Autodesk Inventor part; units mm, degrees
ref_plane "YZ Plane" through (0, 0, 0) normal (1, 0, 0) x (0, 1, 0)
ref_plane "XZ Plane" through (0, 0, 0) normal (0, 1, 0) x (-1, 0, 0)
ref_plane "XY Plane" through (0, 0, 0) normal (0, 0, 1) x (1, 0, 0)
sketch "Sketch1" plane through (0, 0, 0) normal (0, 0, 1) x (1, 0, 0)
  line L0 (0, 8.1389) -> (7.0485, 4.0695)
  line L1 (7.0485, 4.0695) -> (7.0485, -4.0695)
  line L2 (7.0485, -4.0695) -> (0, -8.1389)
  line L3 (0, -8.1389) -> (-7.0485, -4.0695)
  line L4 (-7.0485, -4.0695) -> (-7.0485, 4.0695)
  line L5 (-7.0485, 4.0695) -> (0, 8.1389)
  line L6 (0, 11.3945) -> (0, -11.3945)
  line L7 (-9.8679, 0) -> (9.8679, 0)
  point P0 (0, 0)
  dimension "d0" = 14.097
extrude "Extrusion1" add sketch "Sketch1" along normal blind 11.6332
sketch "Sketch2" plane through (0, 0, 0) normal (1, 0, 0) x (0, 1, 0)
  line L0 (8.1389, 0) -> (8.1389, 11.6332)
  line L1 (4.0695, 11.6332) -> (-4.0695, 11.6332)
  line L2 (8.1389, 11.6332) -> (4.0695, 11.6332)
  line L3 (4.0695, 11.6332) -> (8.1389, 11.6332)
  line L4 (-4.0695, 11.6332) -> (4.0695, 11.6332)
  line L5 (-8.1389, 11.6332) -> (-4.0695, 11.6332)
  line L6 (-4.0695, 11.6332) -> (-8.1389, 11.6332)
  line L7 (8.1389, 7.4422) -> (6.5913, 8.9898)
  line L8 (6.5913, 8.9898) -> (6.5913, 11.6332)
  line L9 (8.1389, 11.6332) -> (8.1389, 7.4422)
  line L10 (6.223, 11.2522) -> (3.683, 11.2522)
  line L11 (3.683, 11.2522) -> (3.683, 8.7122)
  line L12 (3.683, 8.7122) -> (6.223, 8.7122)
  line L13 (6.223, 8.7122) -> (6.223, 11.2522)
  line L14 (0, 18.0282) -> (0, -3.0895)
  arc A0 (7.0485, 0) -> (8.1389, 0.762) centre (6.1895, 2.3903) ccw
  line L15 (8.1389, 0) -> (4.0695, 0)
  line L16 (7.0485, 0) -> (8.1389, 0)
  line L17 (8.1389, 0.762) -> (8.1389, 0)
  dimension "d3" = 4.191
  dimension "d4" = 45
  dimension "d5" = 6.5913
  dimension "d6" = 3.683
  dimension "d7" = 0.381
  dimension "d8" = 2.54
  dimension "d9" = 2.54
  dimension "d11" = 7.0485
  dimension "d12" = 0.762
  dimension "d13" = 2.54
revolve "Revolution1" cut sketch "Sketch2" angle 360 about axis through (0, 0, 0) along (0, 0, -1) contours L7 L8 L2 L0
revolve "Revolution2" cut sketch "Sketch2" angle 360 about axis through (0, 0, 0) along (0, 0, -1) contours L15 A0 L0
hole "Hole1" at (0, 0, 11.6332) direction (0, 0, -1) diameter 7.7978 end through all
fillet "Fillet1" radius 0.381 3 edges at (0, -6.5913, 8.9898) (0, -6.5913, 11.6332) (0, 3.8989, 11.6332)
revolve "Revolution3" add sketch "Sketch2" angle 360 about axis through (0, 0, 0) along (0, 0, -1) contours L13 L12 L11 L10
properties part number "HW-00026" material "Steel"
The model under review builds one solid part; all positions refer to its coordinate system, in mm. A direction names the side the tool comes from. Coordinates: 2 decimals unless noted, no trailing zeros. Write each loop counter-clockwise with the first axis right and the second up, starting at its lowest first coordinate (ties: lowest second). Pieces come first, ordered by that corner, then holes. Notation, with made-up numbers: (30.25, -38.75) -> (65.25, -38.75) arc R21 ccw to (65.25, -6.75) -> close; hole circle Ø5 at (36, -38.75). An arc over 180 degrees is marked (long way). Answer in a Markdown table with one row per item.
1. For faces 1 (the cylindrical face through (2.372, 3.094, 4.295)), 2 (the flat face through (-3.57, 6.08, 4.21)), 3 (the cylindrical face through (6.435, -1.429, 10.215)), list the 3-axis set-ups (+Z, -Z, +X, -X, +Y, -Y) from which the entire face can be reached by the end or side of a thin tool; tool diameter is ignored.
Answers below:
| item | result |
|---|---|
| face 1 | -Z |
| face 2 | +Z, -Z, -X, +Y |
| face 3 | +Z |
2. Clearance check with flat-ended pins moving along their axes: pin 1 Ø1 at (x, z) = (2.5, 9.5) entering from -Y; pin 2 Ø3 at (y, z) = (6, 5) entering from +X; pin 3 Ø2 at (x, y) = (-0.5, -1) entering from -Z. State where each tip first meets the part, or that it passes through.
Answers below:
| item | result |
|---|---|
| pin 1 | stops at y = -6.28 |
| pin 2 | stops at x = 6.3 |
| pin 3 | passes through |
3. Wall thickness on probe 1 along X at (y, z) = (0, 5.75); probe 2 along X at (y, z) = (0, 10); probe 3 along Z at (x, y) = (3.75, 0.5): over which ranges is each line inside the solid? List them lowest first. Write a range as [from, to].
Answers below:
| item | result |
|---|---|
| probe 1 | x = [-7.05, -3.9], [3.9, 7.05] |
| probe 2 | x = [-6.59, -3.68], [3.68, 6.59] |
| probe 3 | z = [8.71, 11.25] |
4. We need section A-A, the plane z = 1.5. State the section outline as (x, y) points.
Answers below:
| item | result |
|---|---|
| outline | (-7.05, -4.07) -> (0, -8.14) -> (7.05, -4.07) -> (7.05, 4.07) -> (0, 8.14) -> (-7.05, 4.07) -> close; hole circle Ø7.8 at (0, 0) |
